Geometry check sheet. Reference: drawing and pictorial views, mm from the part's lowest x, y, z. A direction names the side the tool comes from. Give positions to 0.01 mm unless a question says otherwise; leave off trailing zeros. Loops run counter-clockwise (first coordinate to the right, second up) from the corner with the lowest first, then second, coordinate; pieces in that order, holes last. Notation, with made-up numbers: (21.25, 2.25) -> (45.25, 2.25) arc R15 cw to (45.25, 15.25) -> close; hole circle Ø7 at (26.25, -4.75). An arc over 180 degrees is marked (long way). Answer in a Markdown table with one row per item. Add a question column.
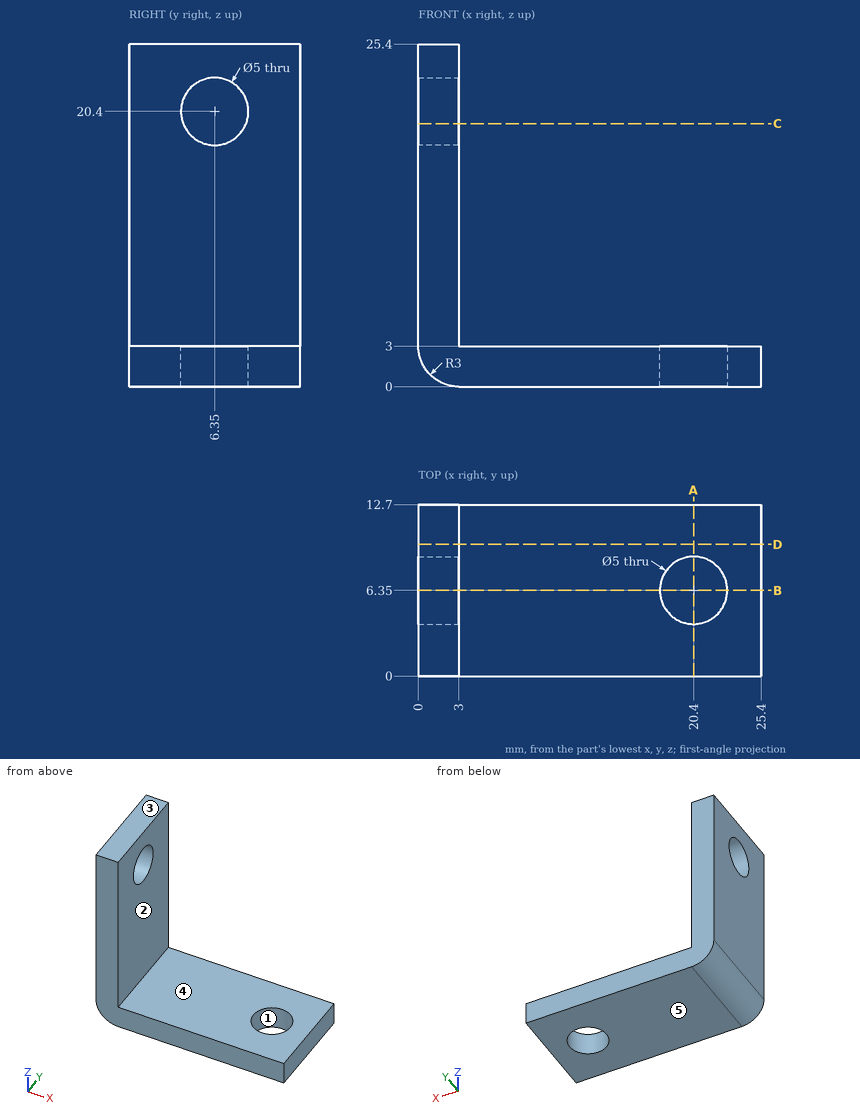
1. Gauge pin test, flat ends, axial feed: pin 1 Ø2 at (y, z) = (10, 6) entering from +X; pin 2 Ø2 at (x, y) = (16.5, 2) entering from +Z. Record the tip position at first contact, or that the pin passes through.
2. Access from +Z, -Z, +X, -X, +Y, -Y to the whole of each face (thin tool, end or side, straight path). Record for the marked faces 4 and 5.
3. Material ranges on L1, parallel to Y at x = 20.4, z = 1.5; L2, parallel to X at y = 10.5, z = 17.25, recorded low to high. Write a range as from..to.
4. Release check for a two-part mould opening along X. For the marked faces 1, 2 and 3 record: released by +X, released by -X, zero draft, split by the parting line, or undercut.
5. Sectioned sample at B-B (y = 6.35). Enter the section's corners in (x, z).
6. Sectioned sample at A-A (x = 20.4). Enter the section's corners in (y, z), plus the area to 3 significant figures.
7. Sectioned sample at C-C (z = 19.5). Enter the section's corners in (x, y).
8. Sectioned sample at D-D (y = 9.75). Enter the section's corners in (x, z).
Response:
| question | item | result |
|---|---|---|
| 1 | pin 1 | stops at x = 3 |
| 1 | pin 2 | stops at z = 3 |
| 2 | face 4 | +Z, +X, +Y, -Y |
| 2 | face 5 | -Z, +X, -X, +Y, -Y |
| 3 | L1 | y = 0..3.85, 8.85..12.7 |
| 3 | L2 | x = 0..3 |
| 4 | face 1 | undercut |
| 4 | face 2 | released by +X |
| 4 | face 3 | zero draft |
| 5 | outline | (0, 3) arc R3 ccw to (3, 0) -> (17.9, 0) -> (17.9, 3) -> (3, 3) -> (3, 17.9) -> (0, 17.9) -> close; (0, 22.9) -> (3, 22.9) -> (3, 25.4) -> (0, 25.4) -> close; (22.9, 0) -> (25.4, 0) -> (25.4, 3) -> (22.9, 3) -> close |
| 6 | outline | (0, 0) -> (3.85, 0) -> (3.85, 3) -> (0, 3) -> close; (8.85, 0) -> (12.7, 0) -> (12.7, 3) -> (8.85, 3) -> close |
| 6 | area | 23.1 mm2 |
| 7 | outline | (0, 0) -> (3, 0) -> (3, 4.02) -> (0, 4.02) -> close; (0, 8.68) -> (3, 8.68) -> (3, 12.7) -> (0, 12.7) -> close |
| 8 | outline | (0, 3) arc R3 ccw to (3, 0) -> (25.4, 0) -> (25.4, 3) -> (3, 3) -> (3, 25.4) -> (0, 25.4) -> close |
